Could you check a few things on this model? Use its own coordinates, in mm. A direction names the side the tool comes from. Give positions to 0.01 mm unless a question says otherwise; leave off trailing zeros. Write each loop counter-clockwise with the first axis right and the second up, starting at its lowest first coordinate (ties: lowest second). Pieces come first, ordered by that corner, then holes. Notation, with made-up numbers: (-34, 81) - (-4, 81) arc R12 ccw to (-4, 95) - close; hole circle Ø9 at (11.5, 28). An arc over 180 degrees is marked (long way). Answer in a Markdown table with one row per item.
Autodesk Inventor part; units mm, degrees
ref_plane "YZ Plane" through (0, 0, 0) normal (1, 0, 0) x (0, 1, 0)
ref_plane "XZ Plane" through (0, 0, 0) normal (0, 1, 0) x (-1, 0, 0)
ref_plane "XY Plane" through (0, 0, 0) normal (0, 0, 1) x (1, 0, 0)
sketch "Sketch1" plane through (0, 0, 0) normal (0, 0, 1) x (1, 0, 0)
  line L0 (-40, -42.5) -> (40, -42.5)
  line L1 (40, -42.5) -> (40, 42.5)
  line L2 (40, 42.5) -> (-40, 42.5)
  line L3 (-40, 42.5) -> (-40, -42.5)
  line L4 (-40, -42.5) -> (40, 42.5) construction
  line L5 (40, -42.5) -> (-40, 42.5) construction
  line L6 (-28.7479, 32.175) -> (28.7479, 32.175) construction
  line L7 (28.7479, 32.175) -> (28.7479, -32.175) construction
  line L8 (28.7479, -32.175) -> (-28.7479, -32.175) construction
  line L9 (-28.7479, -32.175) -> (-28.7479, 32.175) construction
  line L10 (-28.7479, 32.175) -> (28.7479, -32.175) construction
  line L11 (28.7479, 32.175) -> (-28.7479, -32.175) construction
  circle A0 centre (28.7479, -32.175) radius 2.5 construction
  circle A1 centre (-28.7479, -32.175) radius 2.5 construction
  arc A2 (-28.7479, 32.175) -> (-13.7479, 34.175) centre (-28.7479, 89.425) ccw construction
  arc A3 (-28.7479, 29.675) -> (-13.0929, 31.7623) centre (-28.7479, 89.425) ccw construction
  arc A4 (-28.7479, 34.675) -> (-14.403, 36.5877) centre (-28.7479, 89.425) ccw construction
  arc A5 (-28.7479, 34.675) -> (-28.7479, 29.675) centre (-28.7479, 32.175) ccw construction
  arc A6 (-13.0929, 31.7623) -> (-14.403, 36.5877) centre (-13.7479, 34.175) ccw construction
  point P0 (0, 0)
  dimension "d0" = 80
  dimension "d1" = 64.35
  dimension "d2" = 5
  dimension "d3" = 5
  dimension "d4" = 5
  dimension "d5" = 2
  dimension "d6" = 15
  dimension "d7" = 85
extrude "Extrusion1" add sketch "Sketch1" along normal mid plane 6.35
sketch "Sketch2" plane through (0, 0, 3.175) normal (0, 0, 1) x (1, 0, 0)
  line L0 (-40, -42.5) -> (40, -42.5)
  line L1 (-40, 42.5) -> (-40, -42.5)
  line L2 (40, -42.5) -> (40, 42.5)
  point P0 (0, 0)
  point P1 (-32.5, -35)
  point P2 (32.5, -35)
  dimension "d11" = 7.5
  dimension "d12" = 7.5
  dimension "d13" = 7.5
hole "Hole1" at (-32.5, -35, 3.175) at (32.5, -35, 3.175) direction (0, 0, -1) diameter 5.5 end through all
sketch "Sketch3" plane through (0, 0, 3.175) normal (0, 0, 1) x (1, 0, 0)
  circle A0 centre (-32.5, -35) radius 2.75
  circle A1 centre (32.5, -35) radius 2.75
  arc A2 (-32.5, 29) -> (-22.5, 31.5) centre (-32.5, 50.25) ccw construction
  arc A3 (-32.5, 26.25) -> (-21.2059, 29.0735) centre (-32.5, 50.25) ccw
  arc A4 (-32.5, 31.75) -> (-23.7941, 33.9265) centre (-32.5, 50.25) ccw
  arc A5 (-32.5, 31.75) -> (-32.5, 26.25) centre (-32.5, 29) ccw
  arc A6 (-21.2059, 29.0735) -> (-23.7941, 33.9265) centre (-22.5, 31.5) ccw
  line L0 (0, 0) -> (0, 8.7533)
  arc A7 (22.5, 31.5) -> (32.5, 29) centre (32.5, 50.25) ccw construction
  arc A8 (21.2059, 29.0735) -> (32.5, 26.25) centre (32.5, 50.25) ccw
  arc A9 (23.7941, 33.9265) -> (32.5, 31.75) centre (32.5, 50.25) ccw
  arc A10 (32.5, 26.25) -> (32.5, 31.75) centre (32.5, 29) ccw
  arc A11 (23.7941, 33.9265) -> (21.2059, 29.0735) centre (22.5, 31.5) ccw
  dimension "d21" = 64
  dimension "d22" = 2.5
  dimension "d23" = 10
  dimension "d24" = 2.75
extrude "Extrusion2" cut sketch "Sketch3" against normal blind 10 contours A5 A4 A6 A3 | A11 A9 A10 A8
fillet "Fillet1" radius 5 4 edges at (-40, 42.5, 0) (-40, -42.5, 0) (40, 42.5, 0) (40, -42.5, 0)
sketch "Sketch5" plane through (0, 0, 3.175) normal (0, 0, 1) x (1, 0, 0)
  line L0 (-35, 1.95) -> (-32.5, 1.95)
  line L1 (-32.5, 1.95) -> (-32.5, -6.55)
  line L2 (-32.5, -6.55) -> (-35, -6.55)
  line L3 (-35, -6.55) -> (-35, 1.95)
  line L4 (-35, 1.95) -> (-32.5, -6.55) construction
  line L5 (-32.5, 1.95) -> (-35, -6.55) construction
  line L6 (-35, -42.5) -> (35, -42.5)
  line L7 (-40, 37.5) -> (-40, -37.5)
  line L8 (0, 0) -> (0, 7.9941)
  line L9 (35, 1.95) -> (32.5, 1.95)
  line L10 (32.5, 1.95) -> (32.5, -6.55)
  line L11 (32.5, -6.55) -> (35, -6.55)
  line L12 (35, -6.55) -> (35, 1.95)
  line L13 (35, 1.95) -> (32.5, -6.55) construction
  line L14 (32.5, 1.95) -> (35, -6.55) construction
  line L15 (-38, -2.3) -> (-40, -3.4547)
  line L16 (-40, -3.4547) -> (-40, -1.1453)
  line L17 (-40, -1.1453) -> (-38, -2.3)
  line L18 (38, -2.3) -> (40, -3.4547)
  line L19 (40, -3.4547) -> (40, -1.1453)
  line L20 (40, -1.1453) -> (38, -2.3)
  line L21 (-30, 1.95) -> (-27.5, 1.95)
  line L22 (-27.5, 1.95) -> (-27.5, -6.55)
  line L23 (-27.5, -6.55) -> (-30, -6.55)
  line L24 (-30, -6.55) -> (-30, 1.95)
  line L25 (-30, 1.95) -> (-27.5, -6.55) construction
  line L26 (-27.5, 1.95) -> (-30, -6.55) construction
  line L27 (30, 1.95) -> (27.5, 1.95)
  line L28 (27.5, 1.95) -> (27.5, -6.55)
  line L29 (27.5, -6.55) -> (30, -6.55)
  line L30 (30, -6.55) -> (30, 1.95)
  line L31 (30, 1.95) -> (27.5, -6.55) construction
  line L32 (27.5, 1.95) -> (30, -6.55) construction
  line L33 (-22.5, 1.95) -> (-20, 1.95)
  line L34 (-20, 1.95) -> (-20, -6.55)
  line L35 (-20, -6.55) -> (-22.5, -6.55)
  line L36 (-22.5, -6.55) -> (-22.5, 1.95)
  line L37 (-22.5, 1.95) -> (-20, -6.55) construction
  line L38 (-20, 1.95) -> (-22.5, -6.55) construction
  line L39 (20, 1.95) -> (22.5, 1.95)
  line L40 (22.5, 1.95) -> (22.5, -6.55)
  line L41 (22.5, -6.55) -> (20, -6.55)
  line L42 (20, -6.55) -> (20, 1.95)
  line L43 (20, 1.95) -> (22.5, -6.55) construction
  line L44 (22.5, 1.95) -> (20, -6.55) construction
  point P0 (-33.75, -2.3)
  point P1 (33.75, -2.3)
  point P2 (-39.3333, -2.3)
  point P3 (-33.75, -2.3)
  point P4 (39.3333, -2.3)
  point P5 (-40, -1.1453)
  point P6 (-28.75, -2.3)
  point P7 (-28.75, -2.3)
  point P8 (-33.75, -2.3)
  point P9 (28.75, -2.3)
  point P10 (28.75, -2.3)
  point P11 (-21.25, -2.3)
  point P12 (21.25, -2.3)
  dimension "d40" = 2.5
  dimension "d41" = 8.5
  dimension "d42" = 40.2
  dimension "d46" = 2
  dimension "d51" = 5
  dimension "d52" = 5
  dimension "d53" = 5
  dimension "d69" = 10
extrude "Extrusion3" cut sketch "Sketch5" against normal blind 10 contours L21 L22 L23 L24 | L30 L29 L28 L27
sketch "Sketch7" plane through (0, 0, 3.175) normal (0, 0, 1) x (1, 0, 0)
  line L0 (30, 1.95) -> (30, -6.55)
  line L1 (30, -6.55) -> (27.5, -6.55)
  line L2 (27.5, -6.55) -> (27.5, 1.95)
  line L3 (27.5, 1.95) -> (30, 1.95)
  line L4 (-27.5, 1.95) -> (-27.5, -6.55)
  line L5 (-27.5, -6.55) -> (-30, -6.55)
  line L6 (-30, -6.55) -> (-30, 1.95)
  line L7 (-30, 1.95) -> (-27.5, 1.95)
  arc A0 (35, -42.5) -> (40, -37.5) centre (35, -37.5) ccw
  line L8 (40, -37.5) -> (40, 37.5)
  arc A1 (40, 37.5) -> (35, 42.5) centre (35, 37.5) ccw
  line L9 (35, 42.5) -> (-35, 42.5)
  arc A2 (-35, 42.5) -> (-40, 37.5) centre (-35, 37.5) ccw
  line L10 (-40, 37.5) -> (-40, -37.5)
  arc A3 (-40, -37.5) -> (-35, -42.5) centre (-35, -37.5) ccw
  line L11 (-35, -42.5) -> (35, -42.5)
  arc A4 (23.7941, 33.9265) -> (32.5, 31.75) centre (32.5, 50.25) ccw
  arc A5 (32.5, 26.25) -> (32.5, 31.75) centre (32.5, 29) ccw
  arc A6 (21.2059, 29.0735) -> (32.5, 26.25) centre (32.5, 50.25) ccw
  arc A7 (23.7941, 33.9265) -> (21.2059, 29.0735) centre (22.5, 31.5) ccw
  arc A8 (-32.5, 26.25) -> (-21.2059, 29.0735) centre (-32.5, 50.25) ccw
  arc A9 (-32.5, 31.75) -> (-32.5, 26.25) centre (-32.5, 29) ccw
  arc A10 (-32.5, 31.75) -> (-23.7941, 33.9265) centre (-32.5, 50.25) ccw
  arc A11 (-21.2059, 29.0735) -> (-23.7941, 33.9265) centre (-22.5, 31.5) ccw
  circle A12 centre (-32.5, -35) radius 2.75
  circle A13 centre (32.5, -35) radius 2.75
  line L12 (-30, 1.95) -> (-27.5, 1.95)
  line L13 (-30, 1.95) -> (-40, 1.95)
  line L14 (-40, 1.95) -> (-40, -6.55)
  line L15 (-40, -6.55) -> (-30, -6.55)
  line L16 (-30, -6.55) -> (-30, 1.95)
  line L17 (30, -6.55) -> (30, 1.95)
  line L18 (30, 1.95) -> (40, 1.95)
  line L19 (40, 1.95) -> (40, -6.55)
  line L20 (40, -6.55) -> (30, -6.55)
  line L21 (30, -6.55) -> (30, 1.95)
  point P0 (0, 0)
extrude "Extrusion5" cut sketch "Sketch7" against normal blind 1 contours L18 L8 L20 L0 | L13 L6 L15 L10
sketch "Sketch8" plane through (0, 0, 3.175) normal (0, 0, 1) x (1, 0, 0)
  line L0 (-40, 1.95) -> (-30, 1.95)
  line L1 (-40, -6.55) -> (-40, 1.95)
  line L2 (-30, -6.55) -> (-40, -6.55)
  line L3 (-30, 1.95) -> (-30, -6.55)
  line L4 (30, 1.95) -> (40, 1.95)
  line L5 (30, -6.55) -> (30, 1.95)
  line L6 (40, -6.55) -> (30, -6.55)
  line L7 (40, 1.95) -> (40, -6.55)
  circle A0 centre (-35, -2.3) radius 2.5
  circle A1 centre (35, -2.3) radius 2.5
  point P0 (0, 0)
  point P1 (-35, 1.95)
  point P2 (-30, -2.3)
  point P3 (30, -2.3)
  point P4 (35, 1.95)
  dimension "d56" = 5
  dimension "d57" = 5
extrude "Extrusion6" cut sketch "Sketch8" against normal blind 10 contours A0 | A1
sketch "Sketch9" plane through (0, 0, 3.175) normal (0, 0, 1) x (1, 0, 0)
  circle A0 centre (32.5, -35) radius 2.75
  circle A1 centre (-32.5, -35) radius 2.75
  arc A2 (-32.5, 26.25) -> (-21.2059, 29.0735) centre (-32.5, 50.25) ccw
  arc A3 (-32.5, 31.75) -> (-32.5, 26.25) centre (-32.5, 29) ccw
  arc A4 (-32.5, 31.75) -> (-23.7941, 33.9265) centre (-32.5, 50.25) ccw
  arc A5 (-21.2059, 29.0735) -> (-23.7941, 33.9265) centre (-22.5, 31.5) ccw
  arc A6 (23.7941, 33.9265) -> (32.5, 31.75) centre (32.5, 50.25) ccw
  arc A7 (32.5, 26.25) -> (32.5, 31.75) centre (32.5, 29) ccw
  arc A8 (21.2059, 29.0735) -> (32.5, 26.25) centre (32.5, 50.25) ccw
  arc A9 (23.7941, 33.9265) -> (21.2059, 29.0735) centre (22.5, 31.5) ccw
  line L0 (27.5, 1.95) -> (40, 1.95)
  line L1 (40, 1.95) -> (40, 37.5)
  arc A10 (40, 37.5) -> (35, 42.5) centre (35, 37.5) ccw
  line L2 (35, 42.5) -> (-35, 42.5)
  arc A11 (-35, 42.5) -> (-40, 37.5) centre (-35, 37.5) ccw
  line L3 (-40, 37.5) -> (-40, 1.95)
  line L4 (-40, 1.95) -> (-27.5, 1.95)
  line L5 (-27.5, 1.95) -> (-27.5, -6.55)
  line L6 (-27.5, -6.55) -> (-40, -6.55)
  line L7 (-40, -6.55) -> (-40, -37.5)
  arc A12 (-40, -37.5) -> (-35, -42.5) centre (-35, -37.5) ccw
  line L8 (-35, -42.5) -> (35, -42.5)
  arc A13 (35, -42.5) -> (40, -37.5) centre (35, -37.5) ccw
  line L9 (40, -37.5) -> (40, -6.55)
  line L10 (40, -6.55) -> (27.5, -6.55)
  line L11 (27.5, -6.55) -> (27.5, 1.95)
  circle A14 centre (-35, -2.3) radius 2.5
  circle A15 centre (35, -2.3) radius 2.5
  point P0 (0, 0)
  point P1 (-35, 6.2)
  point P2 (-35, -10.8)
  point P3 (35, -10.8)
  point P4 (35, 6.2)
  dimension "d60" = 17
  dimension "d61" = 8.5
hole "Hole3" at (-35, 6.2, 3.175) at (-35, -10.8, 3.175) at (35, -10.8, 3.175) at (35, 6.2, 3.175) direction (0, 0, -1) diameter 5 depth 28.25 tip angle 118
sketch "Sketch10" plane through (0, 0, 3.175) normal (0, 0, 1) x (1, 0, 0)
  line L0 (-20, 20) -> (20, 20) construction
  line L1 (20, 20) -> (20, -20) construction
  line L2 (20, -20) -> (-20, -20) construction
  line L3 (-20, -20) -> (-20, 20) construction
  line L4 (-20, 20) -> (20, -20) construction
  line L5 (20, 20) -> (-20, -20) construction
  line L6 (-10, 31.25) -> (10, 31.25) construction
  line L7 (35, 42.5) -> (-35, 42.5) construction
  line L8 (-10, -31.25) -> (10, -31.25) construction
  line L9 (-32, 18.9) -> (32, 18.9) construction
  line L10 (32, 18.9) -> (32, -24.9) construction
  line L11 (32, -24.9) -> (-32, -24.9) construction
  line L12 (-32, -24.9) -> (-32, 18.9) construction
  line L13 (-32, 18.9) -> (32, -24.9) construction
  line L14 (32, 18.9) -> (-32, -24.9) construction
  point P0 (0, 0)
  point P1 (0, 31.25)
  point P2 (0, 0)
  point P3 (0, -31.25)
  point P4 (0, 0)
  point P5 (0, -3)
  point P6 (0, -3)
  point P7 (34, 18.9)
  point P8 (-21.8, 18.9)
  dimension "d70" = 40
  dimension "d71" = 40
  dimension "d72" = 20
  dimension "d73" = 11.25
  dimension "d74" = 11.25
  dimension "d75" = 11.25
  dimension "d83" = 64
  dimension "d84" = 43.8
  dimension "d85" = 24.9
  dimension "d86" = 2
  dimension "d87" = 10.2
hole "Hole4" at (-21.8, 18.9, 3.175) at (34, 18.9, 3.175) at (32, -24.9, 3.175) at (-32, -24.9, 3.175) direction (0, 0, -1) diameter 5 end through all
sketch "Sketch11" plane through (0, 0, 3.175) normal (0, 0, 1) x (1, 0, 0)
  line L0 (-29.6544, 25.4909) -> (-13.6801, 25.4909)
  line L1 (-13.6801, 25.4909) -> (-13.6801, 10.7062)
  line L2 (-13.6801, 10.7062) -> (-29.6544, 10.7062)
  line L3 (-29.6544, 10.7062) -> (-29.6544, 25.4909)
  point P0 (0, 0)
extrude "Extrusion7" [suppressed]
equation "\"d52\" = d51"
equation "\"d53\" = d52"
equation "\"d74\" = d73"
equation "\"d75\" = d73"
properties part number "x carraige plate new" material "PMMA Plastic"
1) On a 3-axis mill with a long thin cutter (end or side, diameter ignored), from which of +Z, -Z, +X, -X, +Y, -Y can I reach the whole of each face in a straight line? I mean faces 1 (the face through (31.5, 1.95, 2.4)), 2 (the face through (-30, -2, 0)), 3 (the face through (-38.57, 41, -0.04)). Say none if no direction works.
Check values:
| item | result |
|---|---|
| face 1 | +Z |
| face 2 | +Z, -Z |
| face 3 | +Z, -Z, -X, +Y |
2) Imagine slicing it at A-A (y = -10.8). List the corners of the cut face in (x, z) for me (3 decimals).
Check values:
| item | result |
|---|---|
| outline | (-40, -3.175) - (-37.5, -3.175) - (-37.5, 3.175) - (-40, 3.175) - close; (-32.5, -3.175) - (32.5, -3.175) - (32.5, 3.175) - (-32.5, 3.175) - close; (37.5, -3.175) - (40, -3.175) - (40, 3.175) - (37.5, 3.175) - close |
3) Will this pin go through, and if not, where does the flat tip stop? P1, Ø4, axis at x = -35, y = -10.8, coming from the -Z side.
Check values:
| item | result |
|---|---|
| P1 | passes through |
4) We'd pull the mould along Y, two halves only. Please class faces 4 (the face through (31.4, -6.55, 2.4)), 5 (the face through (40, -1, 0)), 6 (the face through (-38.57, -41, 0.04)): +Y half, -Y half, draft (parallel to the pull), parting line (faces both ways), or undercut.
Check values:
| item | result |
|---|---|
| face 4 | undercut |
| face 5 | draft |
| face 6 | -Y half |
5) Imagine slicing it at B-B (y = -2.3). List the corners of the cut face in (x, z) for me (3 decimals).
Check values:
| item | result |
|---|---|
| outline | (-40, -3.175) - (-37.5, -3.175) - (-37.5, 2.175) - (-40, 2.175) - close; (-32.5, -3.175) - (-30, -3.175) - (-30, 2.175) - (-32.5, 2.175) - close; (-27.5, -3.175) - (27.5, -3.175) - (27.5, 3.175) - (-27.5, 3.175) - close; (30, -3.175) - (32.5, -3.175) - (32.5, 2.175) - (30, 2.175) - close; (37.5, -3.175) - (40, -3.175) - (40, 2.175) - (37.5, 2.175) - close |
6) If I drill on line 1 (X direction, y = -35, z = 1.5); line 2 (X direction, y = 18.9, z = -1.25); line 3 (Y direction, x = -35, z = 1.75), over which ranges is the centre line in solid material (lowest first)?
Check values:
| item | result |
|---|---|
| line 1 | x = -40 to -35.25, -29.75 to 29.75, 35.25 to 40 |
| line 2 | x = -40 to -24.3, -19.3 to 31.5, 36.5 to 40 |
| line 3 | y = -42.5 to -36.15, -33.85 to -13.3, -8.3 to -4.8, 0.2 to 3.7, 8.7 to 27.85, 30.15 to 42.5 |
